Verification items for the finished model (mm, model axes). A direction names the side the tool comes from. Give positions to 0.01 mm unless a question says otherwise; leave off trailing zeros. Write each loop counter-clockwise with the first axis right and the second up, starting at its lowest first coordinate (ties: lowest second). Pieces come first, ordered by that corner, then holes. Notation, with made-up numbers: M -31.5,84.25 L -6.5,84.25 A19 cw -6.5,98.25 Z; hole C 43.5,17.5 d3. An arc over 180 degrees is marked long. Answer as a JSON object with one key per item and string values.
Autodesk Inventor part; units mm, degrees
ref_plane "YZ Plane" through (0, 0, 0) normal (1, 0, 0) x (0, 1, 0)
ref_plane "XZ Plane" through (0, 0, 0) normal (0, 1, 0) x (-1, 0, 0)
ref_plane "XY Plane" through (0, 0, 0) normal (0, 0, 1) x (1, 0, 0)
sketch "Sketch1" plane through (0, 0, 0) normal (0, 0, 1) x (1, 0, 0)
  line L0 (-5, -10) -> (5, -10)
  line L1 (5, -10) -> (5, 10)
  line L2 (5, 10) -> (-5, 10)
  line L3 (-5, 10) -> (-5, -10)
  line L4 (-5, -10) -> (5, 10) construction
  line L5 (5, -10) -> (-5, 10) construction
  circle A0 centre (-10.5904, 5.4479) radius 1.6
  circle A1 centre (-8.5404, 5.4479) radius 0.75
  point P0 (0, 0)
  point P1 (-9.0782, 4.9252)
  point P2 (-9.0782, 5.9707)
  dimension "d0" = 3.2
  dimension "d1" = 2.05
  dimension "d2" = 1.5
  dimension "d29" = 10
  dimension "d30" = 20
extrude "Extrusion1" add sketch "Sketch1" along normal blind 6 contours L3 L2 L1 L0
sketch "Sketch2" plane through (0, 0, 6) normal (0, 0, 1) x (1, 0, 0)
  circle A0 centre (0, 4.575) radius 1.575
  line L0 (0, 4.575) -> (0, 6.625)
  circle A1 centre (0, 6.625) radius 0.75
  circle A2 centre (-1.7754, 3.55) radius 0.75
  circle A3 centre (1.7754, 3.55) radius 0.75
  line L1 (0, 0) -> (0, 3)
  circle A4 centre (0, -3) radius 2.15
  line L2 (0, -3) -> (0, -5.8)
  circle A5 centre (0, -5.8) radius 1
  circle A6 centre (2.4249, -1.6) radius 1
  circle A7 centre (-2.4249, -1.6) radius 1
  point P0 (1.0418, 3.3938)
  point P1 (1.5439, 4.2634)
  point P2 (0.5021, 6.0678)
  point P3 (-0.5021, 6.0678)
  point P4 (-1.5439, 4.2634)
  point P5 (-1.0418, 3.3938)
  point P6 (-1.4437, -1.4068)
  point P7 (-2.1016, -2.5463)
  point P8 (-0.6579, -5.0469)
  point P9 (0.6579, -5.0469)
  point P10 (2.1016, -2.5463)
  point P11 (1.4437, -1.4068)
  dimension "d5" = 3.15
  dimension "d6" = 2.05
  dimension "d7" = 1.5
  dimension "d10" = 360
  dimension "d17" = 3
  dimension "d18" = 4.3
  dimension "d19" = 2.8
  dimension "d20" = 2
  dimension "d21" = 3
  dimension "d24" = 360
extrude "Extrusion2" cut sketch "Sketch2" against normal blind 10 contours A0 A3 A2 A1 | A4 A5 A7 A6
chamfer "Chamfer1" distance 0.25 angle 80 3 edges at (0, 5.875, 6) (-1.1258, 3.925, 6) (1.1258, 3.925, 6) measured on face at (-4.0339, -0.8488, 6)
chamfer "Chamfer2" distance 0.25 angle 80 3 edges at (-1.5588, -2.1, 6) (1.5588, -2.1, 6) (0, -4.8, 6) measured on face at (-4.0339, -0.8488, 6)
properties part number "Tolerance_test"
1) Access from +Z, -Z, +X, -X, +Y, -Y to the whole of each face (thin tool, end or side, straight path). Record for faces 1 (the face through (0, 10, 3)), 2 (the face through (-1.122, 3.918, 2.323)), 3 (the face through (-0.009, -4.923, 5.281)).
Completed:
{"face 1": "+Z, -Z, +X, -X, +Y", "face 2": "+Z, -Z", "face 3": "+Z"}
2) Section check A-A on y = 5. Record the boundary of the cut face in (x, z), and give its area (3 significant figures).
Completed:
{"outline": "M -5,0 L -1.52,0 L -1.52,6 L -5,6 Z; M 1.52,0 L 5,0 L 5,6 L 1.52,6 Z", "area": "41.8 mm2"}
3) Section check C-C on z = 2. Record the boundary of the cut face in (x, y) (3 decimals), and give its area (3 significant figures).
Completed:
{"outline": "M -5,-10 L 5,-10 L 5,10 L -5,10 Z; hole M -2.102,-2.546 A2.15 ccw -0.658,-5.047 A1 cw 0.658,-5.047 A2.15 ccw 2.102,-2.546 A1 cw 1.444,-1.407 A2.15 ccw -1.444,-1.407 A1 cw Z; hole M -1.544,4.263 A0.75 cw -1.042,3.394 A1.575 ccw 1.042,3.394 A0.75 cw 1.544,4.263 A1.575 ccw 0.502,6.068 A0.75 cw -0.502,6.068 A1.575 ccw Z", "area": "179 mm2"}
4) Release check for a two-part mould opening along X. For faces 4 (the face through (5, 0, 3)), 5 (the face through (0, 3, 3)), 6 (the face through (0, -10, 3)) record: pulls with the +X half, pulls with the -X half, needs draft (parallel to the pull), parting line crosses it, or undercut.
Completed:
{"face 4": "pulls with the +X half", "face 5": "undercut", "face 6": "needs draft"}
5) Thickness scan on L1, parallel to X at y = 6, z = 3.5; L2, parallel to Y at x = -0.25, z = 3.75; L3, parallel to Y at x = 0.75, z = 5.75. Record the ranges inside material, lowest first.
Completed:
{"L1": "x = -5 to -0.67, -0.41 to 0.41, 0.67 to 5", "L2": "y = -10 to -4.83, -0.86 to 3.02, 5.92 to 10", "L3": "y = -10 to -5.01, -0.99 to 3.19, 5.96 to 10"}
6) Section check B-B on z = 5.5. Record the boundary of the cut face in (x, y) (3 decimals).
Completed:
{"outline": "M -5,-10 L 5,-10 L 5,10 L -5,10 Z; hole M -2.049,-2.349 A2.15 ccw -0.461,-5.1 A0.838 cw 0.461,-5.1 A2.15 ccw 2.049,-2.349 A0.838 cw 1.588,-1.551 A2.15 ccw -1.588,-1.551 A0.838 cw Z; hole M -1.49,4.064 A0.588 cw -1.187,3.54 A1.575 ccw 1.187,3.54 A0.588 cw 1.49,4.064 A1.575 ccw 0.303,6.121 A0.588 cw -0.303,6.121 A1.575 ccw Z"}
7) Go/stop test with a flat-tipped pin: pin 1 (5 mm diameter, centred on x = 1.5, y = -1, fed in from -Z). Record where the tip stops, or that it passes through.
Completed:
{"pin 1": "stops at z = 0"}
